Source: CAD feature listing. Evaluate the final solid. Frame: model axes, mm. Give positions to 0.01 mm unless a question says otherwise; leave off trailing zeros. Order: outer loops, then holes, each group sorted by start corner. A loop starts at its lowest first (then second) coordinate and runs counter-clockwise, first axis right, second up.
1) First-contact query: P1, Ø3, axis at x = 2, z = 28, coming from the +Y side; P2, Ø5, axis at x = -2.5, z = -18, coming from the -Y side; P3, Ø1.5, axis at y = 7.5, z = 7, coming from the +X side. Flat tips, straight axial feed; report the tip coordinate or a pass-through.
2) Section C-C, the plane x = 0. Return loops of the section in (y, z), plus the area to 3 significant figures.
3) Material intervals for line 1 (X direction, y = 7.2, z = 0); line 2 (Z direction, x = 0, y = 5); line 3 (Z direction, x = 3, y = 1.5), sorted ascending.
4) Section D-D, the plane z = 0. Return loops of the section in (x, y), plus the area to 3 significant figures.
5) Section B-B, the plane z = 29. Return loops of the section in (x, y), plus the area to 3 significant figures.
6) Section A-A, the plane y = 1.75. Return loops of the section in (x, z), plus the area to 3 significant figures.
Autodesk Inventor part; units mm, degrees
ref_plane "YZ Plane" through (0, 0, 0) normal (1, 0, 0) x (0, 1, 0)
ref_plane "XZ Plane" through (0, 0, 0) normal (0, 1, 0) x (-1, 0, 0)
ref_plane "XY Plane" through (0, 0, 0) normal (0, 0, 1) x (1, 0, 0)
sketch "Boceto1" plane through (0, 0, 0) normal (0, 1, 0) x (-1, 0, 0)
  line L0 (-36, 36) -> (36, 36)
  line L1 (36, 36) -> (36, -36)
  line L2 (36, -36) -> (-36, -36)
  line L3 (-36, -36) -> (-36, 36)
  line L4 (-36, 36) -> (36, -36) construction
  line L5 (36, 36) -> (-36, -36) construction
  line L6 (-34.5, 34.5) -> (34.5, 34.5)
  line L7 (34.5, 34.5) -> (34.5, -34.5)
  line L8 (34.5, -34.5) -> (-34.5, -34.5)
  line L9 (-34.5, -34.5) -> (-34.5, 34.5)
  line L10 (-34.5, 34.5) -> (34.5, -34.5) construction
  line L11 (34.5, 34.5) -> (-34.5, -34.5) construction
  point P0 (0, 0)
  dimension "d0" = 72
  dimension "d1" = 72
  dimension "d2" = 69
  dimension "d3" = 69
extrude "Extrusión1" add sketch "Boceto1" along normal blind 3
sketch "Boceto2" plane through (0, 3, 0) normal (0, 1, 0) x (1, 0, 0)
  line L0 (-36, 36) -> (-36, -36)
  line L1 (-36, -36) -> (36, -36)
  line L2 (36, 36) -> (-36, 36)
  line L3 (36, -36) -> (36, 36)
  line L4 (36, -36) -> (-36, -36)
  line L5 (-36, -36) -> (-36, 36)
  line L6 (-36, 36) -> (36, 36)
  line L7 (36, 36) -> (36, -36)
  line L8 (36, -36) -> (-36, 36) construction
  line L9 (-36, -36) -> (36, 36) construction
  point P0 (0, 0)
extrude "Extrusión2" add sketch "Boceto2" along normal blind 3
sketch "Boceto3" plane through (0, 6, 0) normal (0, 1, 0) x (1, 0, 0)
  line L0 (-36, 36) -> (-36, -36)
  line L1 (-36, -36) -> (36, -36)
  line L2 (36, -36) -> (36, 36)
  line L3 (36, 36) -> (-36, 36)
  circle A0 centre (0, -29) radius 2.5
  circle A1 centre (0, 0) radius 8.5
  circle A2 centre (0, 0) radius 9.5
  line L4 (6, -13) -> (-6, -5) construction
  line L5 (-6, -13) -> (6, -5) construction
  line L6 (-6, -7.3655) -> (-6, -6.0208)
  line L7 (6, -7.3655) -> (6, -6.0208)
  arc A3 (-6, -6.0208) -> (6, -6.0208) centre (0, 0) ccw
  arc A4 (-6, -7.3655) -> (6, -7.3655) centre (0, 0) ccw
  point P0 (0, -9)
  dimension "d8" = 5
  dimension "d9" = 17
  dimension "d10" = 19
extrude "Extrusión3" add sketch "Boceto3" along normal blind 3 contours A1 L6 A2 L7 picked at (9.0782, 0.7435)
sketch "Boceto4" plane through (0, 6, 0) normal (0, 1, 0) x (1, 0, 0)
  circle A0 centre (0, -29) radius 2.5
  point P0 (0, 0)
  dimension "d13" = 5
extrude "Extrusión4" cut sketch "Boceto4" against normal blind 3
properties part number "Tapapotenciometro_v1"
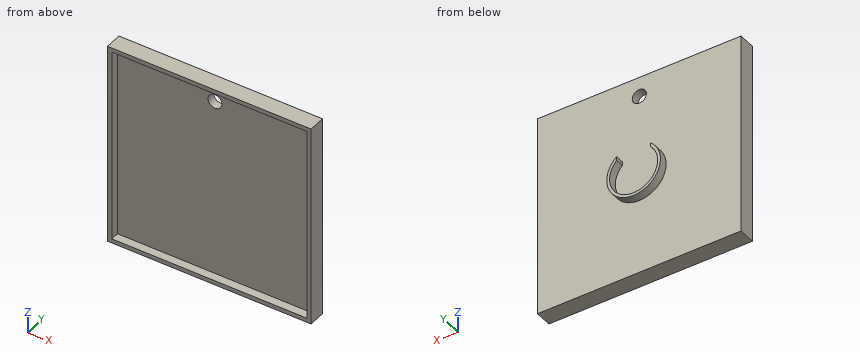
From the geometry:
1. P1: stops at y = 6
1. P2: stops at y = 3
1. P3: stops at x = 7.15
2. outline: (0, -36) - (6, -36) - (6, -9.5) - (9, -9.5) - (9, -8.5) - (6, -8.5) - (6, 26.5) - (3, 26.5) - (3, -34.5) - (0, -34.5) - close; (0, 34.5) - (3, 34.5) - (3, 31.5) - (6, 31.5) - (6, 36) - (0, 36) - close
2. area: 213 mm2
3. line 1: x = -9.5 to -8.5, 8.5 to 9.5
3. line 2: z = -36 to 26.5, 31.5 to 36
3. line 3: z = -36 to -34.5, 34.5 to 36
4. outline: (-36, 0) - (-34.5, 0) - (-34.5, 3) - (34.5, 3) - (34.5, 0) - (36, 0) - (36, 6) - (9.5, 6) - (9.5, 9) - (8.5, 9) - (8.5, 6) - (-8.5, 6) - (-8.5, 9) - (-9.5, 9) - (-9.5, 6) - (-36, 6) - close
4. area: 231 mm2
5. outline: (-36, 0) - (-34.5, 0) - (-34.5, 3) - (-2.5, 3) - (-2.5, 6) - (-36, 6) - close; (2.5, 3) - (34.5, 3) - (34.5, 0) - (36, 0) - (36, 6) - (2.5, 6) - close
5. area: 210 mm2
6. outline: (-36, -36) - (36, -36) - (36, 36) - (-36, 36) - close; hole (-34.5, -34.5) - (34.5, -34.5) - (34.5, 34.5) - (-34.5, 34.5) - close
6. area: 423 mm2
